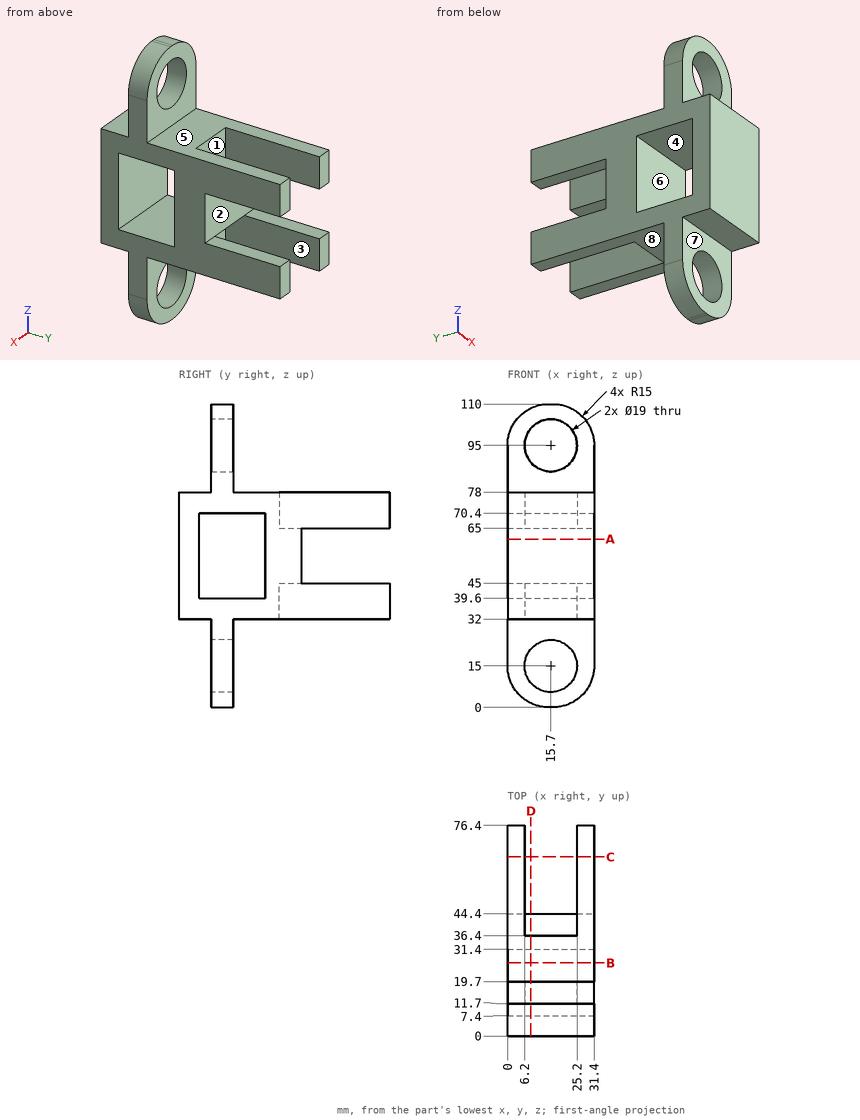
For this review, use the dimensioned drawing (mm, ordinates from the lowest corner) and the shaded views. A direction names the side the tool comes from. Round coordinates to 2 decimals unless told otherwise and drop trailing zeros. Write each loop counter-clockwise with the first axis right and the second up, starting at its lowest first coordinate (ties: lowest second). Pieces come first, ordered by that corner, then holes. Notation, with made-up numbers: (5, 65) - (54, 65) arc R25 cw to (54, 88) - close; hole circle Ø2 at (11, -40). An arc over 180 degrees is marked (long way). One line per item, written item: value. Start each with the question number.
1. Machinability: for the marked faces 1, 2, 3, 4 and 5, which of the approach directions +Z, -Z, +X, -X, +Y, -Y give a long, thin tool a straight path to every point of the face, cutting with its end or side? Answer none if there is none.
2. Consider section C-C on y = 65. Write out the cut boundary in (x, z), and give its area (3 significant figures).
3. To check wall thickness, follow L1, parallel to Z at x = 15, y = 17; L2, parallel to X at y = 73, z = 74.5; L3, parallel to Z at x = 9.5, y = 9. State the ranges of each line that lie inside material, in increasing order. Write a range as from..to.
4. Consider section A-A on z = 61. Write out the cut boundary in (x, y), and give its area (3 significant figures).
5. Consider section B-B on y = 26.5. Write out the cut boundary in (x, z).
6. Clearance check with flat-ended pins moving along their axes: P1, Ø4, axis at x = 18, y = 38.5, coming from the -Z side; P2, Ø9.5, axis at x = 10, y = 8, coming from the -Z side; P3, Ø5, axis at x = 4.5, y = 61, coming from the +Z side; P4, Ø11.5, axis at x = 15.7, z = 95, coming from the +Y side. State where each tip first meets the part, or that it passes through.
7. The part is to be moulded in two halves that separate along Y. For the marked faces 6, 7 and 8, say which applies: released by +Y, released by -Y, zero draft, split by the parting line, or undercut.
8. Consider section D-D on x = 8.5. Write out the cut boundary in (y, z).
Checks:
1. face 1: +Z, +Y
1. face 2: +X, -X, +Y
1. face 3: -Z, +Y
1. face 4: +X, -X
1. face 5: +Z, +X, -X, +Y
2. outline: (0, 32) - (6.2, 32) - (6.2, 45) - (0, 45) - close; (0, 65) - (6.2, 65) - (6.2, 78) - (0, 78) - close; (25.2, 32) - (31.4, 32) - (31.4, 45) - (25.2, 45) - close; (25.2, 65) - (31.4, 65) - (31.4, 78) - (25.2, 78) - close
2. area: 322 mm^2
3. L1: z = 0..5.53, 24.47..39.6, 70.4..85.53, 104.47..110
3. L2: x = 0..6.2, 25.2..31.4
3. L3: z = 32..39.6, 70.4..78
4. outline: (0, 0) - (31.4, 0) - (31.4, 7.4) - (0, 7.4) - close; (0, 31.4) - (31.4, 31.4) - (31.4, 44.4) - (0, 44.4) - close
4. area: 641 mm^2
5. outline: (0, 32) - (31.4, 32) - (31.4, 39.6) - (0, 39.6) - close; (0, 70.4) - (31.4, 70.4) - (31.4, 78) - (0, 78) - close
6. P1: stops at z = 45
6. P2: stops at z = 0.14
6. P3: stops at z = 78
6. P4: passes through
7. face 6: undercut
7. face 7: released by -Y
7. face 8: zero draft
8. outline: (0, 32) - (11.7, 32) - (11.7, 21.2) - (19.7, 21.2) - (19.7, 32) - (36.4, 32) - (36.4, 45) - (44.4, 45) - (44.4, 65) - (36.4, 65) - (36.4, 78) - (19.7, 78) - (19.7, 88.8) - (11.7, 88.8) - (11.7, 78) - (0, 78) - close; (11.7, 1.48) - (19.7, 1.48) - (19.7, 8.8) - (11.7, 8.8) - close; (11.7, 101.2) - (19.7, 101.2) - (19.7, 108.52) - (11.7, 108.52) - close; hole (7.4, 39.6) - (31.4, 39.6) - (31.4, 70.4) - (7.4, 70.4) - close
